For this review, take the finished solid that the model builds, in its own axes (mm). A direction names the side the tool comes from. Round coordinates to 2 decimals unless told otherwise and drop trailing zeros. Order: outer loops, then holes, each group sorted by start corner. A loop starts at its lowest first (then second) coordinate and runs counter-clockwise, first axis right, second up. Notation, with made-up numbers: M -17.75,6 L 19.25,6 A23 cw 19.25,29 Z; hole C 86.5,88 d9. An arc over 180 degrees is marked long. Answer as a JSON object with one key per item and string values.
Autodesk Inventor part; units mm, degrees
ref_plane "YZ Plane" through (0, 0, 0) normal (1, 0, 0) x (0, 1, 0)
ref_plane "XZ Plane" through (0, 0, 0) normal (0, 1, 0) x (-1, 0, 0)
ref_plane "XY Plane" through (0, 0, 0) normal (0, 0, 1) x (1, 0, 0)
sketch "Sketch1" plane through (0, 0, 0) normal (1, 0, 0) x (0, 1, 0)
  line L0 (0, 0) -> (101.6, 0)
  line L1 (101.6, 0) -> (101.6, -94.996)
  line L2 (101.6, -94.996) -> (0, -94.996)
  line L3 (0, -94.996) -> (0, 0)
  dimension "d0" = 101.6
  dimension "d1" = 94.996
extrude "Extrusion1" add sketch "Sketch1" along normal blind 8
sketch "Sketch2" plane through (0, 0, -94.996) normal (0, -1, 0) x (1, 0, 0)
  line L0 (0, 0) -> (0, 94.996)
  line L1 (8, 0) -> (8, 94.996)
  circle A0 centre (4, 72.498) radius 2
  circle A1 centre (4, 22.498) radius 2
  dimension "d6" = 4
extrude "Extrusion2" cut sketch "Sketch2" against normal blind 8
sketch "Sketch3" plane through (8, 0, 0) normal (1, 0, 0) x (0, 0, -1)
  line L0 (0, 101.6) -> (0, 0)
  line L1 (94.996, 101.6) -> (0, 101.6)
  circle A0 centre (47.498, 50.8) radius 4
  dimension "d9" = 8
extrude "Extrusion3" cut sketch "Sketch3" against normal through all
fillet "Fillet1" radius 40.25 2 edges at (4, 101.6, 0) (4, 101.6, -94.996)
properties part number "Base_Attachment"
1) Machinability: for faces 4 (the cylindrical face through (3.57, 3.94, -74.45)), 5 (the flat face through (4, 31, -94.996)), which of the approach directions +Z, -Z, +X, -X, +Y, -Y give a long, thin tool a straight path to every point of the face, cutting with its end or side? Answer none if there is none.
Geometry check:
{"face 4": "-Y", "face 5": "-Z, +X, -X, +Y, -Y"}
2) Mouldability with a two-part tool opening along Z and no side actions: class faces 1 (the cylindrical face through (3.74, 3.944, -20.515)), 2 (the flat face through (8, 39, -47)), 3 (the cylindrical face through (4.06, 90.12, -12.1)) as +Z half, -Z half, draft (parallel to the pull), parting line (faces both ways), or undercut.
Geometry check:
{"face 1": "undercut", "face 2": "draft", "face 3": "+Z half"}
3) Insertion check: P1, Ø4, axis at y = 28.5, z = -58.5, coming from the -X side; P2, Ø1.2, axis at x = 3, z = -22, coming from the -Y side; P3, Ø3, axis at x = 4, z = -72.498, coming from the +Y side; P4, Ø1, axis at x = 4, z = -22.5, coming from the +Y side. Each pin has a flat end and moves straight along its axis. Give the tip position at first contact, or say it passes through.
Geometry check:
{"P1": "stops at x = 0", "P2": "stops at y = 8", "P3": "stops at y = 98.17", "P4": "stops at y = 97.72"}
4) Add section D-D on z = -6. State the section outline as (x, y) points.
Geometry check:
{"outline": "M 0,0 L 8,0 L 8,82.49 L 0,82.49 Z"}
5) Add section C-C on z = -48. State the section outline as (x, y) points.
Geometry check:
{"outline": "M 0,0 L 8,0 L 8,46.83 L 0,46.83 Z; M 0,54.77 L 8,54.77 L 8,101.6 L 0,101.6 Z"}
6) For L1, parallel to Z at x = 4, y = 5; L2, parallel to Z at x = 4.5, y = 49.5; L3, parallel to Y at x = 4, z = -47, list the stretches that pass through material, from the lowest coordinate up.
Geometry check:
{"L1": "z = -95 to -74.5, -70.5 to -24.5, -20.5 to 0", "L2": "z = -95 to -51.28, -43.72 to 0", "L3": "y = 0 to 46.83, 54.77 to 101.6"}
7) Add section B-B on x = 4. State the section outline as (y, z) points.
Geometry check:
{"outline": "M 0,-95 L 61.35,-95 A40.25 ccw 101.6,-54.75 L 101.6,-40.25 A40.25 ccw 61.35,0 L 0,0 L 0,-20.5 L 8,-20.5 L 8,-24.5 L 0,-24.5 L 0,-70.5 L 8,-70.5 L 8,-74.5 L 0,-74.5 Z; hole C 50.8,-47.5 d8"}
8) Add section A-A on y = 50.8. State the section outline as (x, z) points, and give its area (3 significant figures).
Geometry check:
{"outline": "M 0,-95 L 8,-95 L 8,-51.5 L 0,-51.5 Z; M 0,-43.5 L 8,-43.5 L 8,0 L 0,0 Z", "area": "696 mm²"}
